Verification items for the finished model (mm, model axes). A direction names the side the tool comes from. Round coordinates to 2 decimals unless told otherwise and drop trailing zeros. Order: outer loops, then holes, each group sorted by start corner. A loop starts at its lowest first (then second) coordinate and runs counter-clockwise, first axis right, second up. Notation, with made-up numbers: M 58.25,-31 L 92.25,-31 A25 ccw 92.25,-3 Z; hole C 40.25,-25 d9. An arc over 180 degrees is marked long. Return JSON: item names as keys, results as strings. Group by question number.
from build123d import *

# Parameters (mm, degrees)
CROQUIS1_R              = 23.4
CROQUIS1_R_2            = 18.4
SALIENTE_EXTRUIR1_DEPTH = 114
CROQUIS2_R              = 23.4
CROQUIS2_R_2            = 7.5
CROQUIS2_R_3            = 1.25
SALIENTE_EXTRUIR2_DEPTH = 5
CORTAR_EXTRUIR1_DEPTH   = 23.5
CROQUIS6_R              = 11.5
CORTAR_EXTRUIR2_DEPTH   = 2.5
CROQUIS9_R              = 2
SALIENTE_EXTRUIR3_DEPTH = 10
REDONDEO3_R             = 10
CROQUIS10_W             = 23.154362093
CROQUIS10_H             = 20
CORTAR_EXTRUIR3_DEPTH   = 10
SALIENTE_EXTRUIR4_DEPTH = 22
REDONDEO1_R             = 10
CROQUIS12_R             = 18.4
CORTAR_EXTRUIR4_DEPTH   = 78


with BuildPart() as part:
    # Croquis1 → Saliente-Extruir1 (new body)
    with BuildSketch(Plane(origin=(0, 0, 0), x_dir=(0, 0, -1), z_dir=(1, 0, 0))):
        Circle(CROQUIS1_R)
        Circle(CROQUIS1_R_2, mode=Mode.SUBTRACT)
    extrude(amount=SALIENTE_EXTRUIR1_DEPTH)

    # Croquis2 → Saliente-Extruir2 (add)
    with BuildSketch(Plane.ZY):
        Circle(CROQUIS2_R)
        Circle(CROQUIS2_R_2, mode=Mode.SUBTRACT)
        with Locations((-11.138131171, -8.481865008)):
            Circle(CROQUIS2_R_3, mode=Mode.SUBTRACT)
        with Locations((8.481865008, -11.138131171)):
            Circle(CROQUIS2_R_3, mode=Mode.SUBTRACT)
        with Locations((11.138131171, 8.481865008)):
            Circle(CROQUIS2_R_3, mode=Mode.SUBTRACT)
        with Locations((-8.481865008, 11.138131171)):
            Circle(CROQUIS2_R_3, mode=Mode.SUBTRACT)
    extrude(amount=-SALIENTE_EXTRUIR2_DEPTH)

    # Croquis4 → Cortar-Extruir1 (cut, symmetric)
    with BuildSketch(Plane.XY):
        Polygon((114, 0.1), (74, -23.4), (114, -23.4), align=None)
    extrude(amount=CORTAR_EXTRUIR1_DEPTH, both=True, mode=Mode.SUBTRACT)

    # Croquis6 → Cortar-Extruir2 (cut)
    with BuildSketch(Plane(origin=(5, 0, 0), x_dir=(0, 0, -1), z_dir=(1, 0, 0))):
        Circle(CROQUIS6_R)
    extrude(amount=-CORTAR_EXTRUIR2_DEPTH, mode=Mode.SUBTRACT)



with BuildPart() as body_2:
    # Croquis9 → Saliente-Extruir3 (new body, symmetric)
    with BuildSketch(Plane.XY):
        Polygon((73.650159213, -43.69341218), (73.650159213, -63.69341218), (53.650159213, -63.69341218), (53.650159213, -43.69341218), (37, -23.4), (59, -23.4), align=None)
        with Locations((58.650159213, -48.69341218)):
            Circle(CROQUIS9_R, mode=Mode.SUBTRACT)
        with Locations((58.650159213, -58.69341218)):
            Circle(CROQUIS9_R, mode=Mode.SUBTRACT)
        with Locations((68.650159213, -58.69341218)):
            Circle(CROQUIS9_R, mode=Mode.SUBTRACT)
        with Locations((68.650159213, -48.69341218)):
            Circle(CROQUIS9_R, mode=Mode.SUBTRACT)
    extrude(amount=SALIENTE_EXTRUIR3_DEPTH, both=True)

    # Redondeo3
    redondeo3_edges = [body_2.edges().sort_by_distance(p)[0] for p in [
        (53.650159213, -43.69341218, 0),
        (73.650159213, -43.69341218, 0),
    ]]
    fillet(redondeo3_edges, radius=REDONDEO3_R)

    # Croquis10 → Cortar-Extruir3 (cut)
    with BuildSketch(Plane.XY.offset(10)):
        with Locations((62.072978167, -53.69341218)):
            Rectangle(CROQUIS10_W, CROQUIS10_H)
    extrude(amount=-CORTAR_EXTRUIR3_DEPTH, mode=Mode.SUBTRACT)


with BuildPart() as part_1:
    add(part.part)

    add(body_2.part)  # Saliente-Extruir4 merges body 2
    # Croquis11 → Saliente-Extruir4 (add)
    with BuildSketch(Plane(origin=(37, 0, 0), x_dir=(0, 0, -1), z_dir=(1, 0, 0))):
        with BuildLine():
            Line((-10, -23.4), (10, -23.4))
            ThreePointArc((10, -23.4), (0, 25.447200239), (-10, -23.4))
        make_face()
    extrude(amount=SALIENTE_EXTRUIR4_DEPTH)

    # Redondeo1
    redondeo1_edges = [part_1.edges().sort_by_distance(p)[0] for p in [
        (48, -23.4, -10),
        (48, -23.4, 10),
    ]]
    fillet(redondeo1_edges, radius=REDONDEO1_R)

    # Croquis12 → Cortar-Extruir4 (cut, through all)
    with BuildSketch(Plane.ZY.offset(-37)):
        Circle(CROQUIS12_R)
    extrude(amount=-CORTAR_EXTRUIR4_DEPTH, mode=Mode.SUBTRACT)


solid = part_1.part
1. Cross-section at D-D (y = 15.5). Enter the section's corners in (x, z).
2. Cross-section at A-A (z = -3). Give the number of separate pieces and of enclosed holes in the cut face, plus the area to 3 significant figures.
3. Cross-section at B-B (z = 22). Enter the section's corners in (x, y), plus the area to 3 significant figures.
4. Access from +Z, -Z, +X, -X, +Y, -Y to the whole of each face (thin tool, end or side, straight path). Record for faces 4 (the face through (18.241, -22.844, 5.073)), 5 (the face through (58, -36, 10)), 6 (the face through (3.8, 11.4, 1.5)).
5. Draft check along X on faces 1 (the face through (56.65, -58.61, -5.07)), 2 (the face through (1.232, 0.33, -7.493)), 3 (the face through (2.5, 0, -8)). Enter one of: +X half, -X half, draft (parallel to the pull), parting line (faces both ways), or undercut.
6. Thickness scan on line 1 along Y through (x, z) = (11, 0.5); line 2 along Z through (x, y) = (15, 0); line 3 along Z through (x, y) = (65.5, -44.5). Record the ranges inside material, lowest first. Write a range as from..to.
7. Go/stop test with flat-tipped pins: pin 1 (8 mm diameter, centred on x = 62, z = 5.5, fed in from -Y); pin 2 (4.5 mm diameter, centred on x = 68.65, y = -58.69, fed in from -Z); pin 3 (1.5 mm diameter, centred on x = 27, z = 5, fed in from -Y). Record where each tip stops, or that it passes through.
8. Cross-section at C-C (x = 11). Enter the section's corners in (y, z), plus the area to 3 significant figures.
Computed:
{
 "1": {"outline": "M 0,-17.53 L 37,-17.53 L 37,-20.18 L 59,-20.18 L 59,-17.53 L 114,-17.53 L 114,-9.92 L 5,-9.92 L 5,9.92 L 114,9.92 L 114,17.53 L 59,17.53 L 59,20.18 L 37,20.18 L 37,17.53 L 0,17.53 Z"},
 "2": {"separate pieces": "2", "enclosed holes": "4", "area": "1,890 mm²"},
 "3": {"outline": "M 0,-7.97 L 37,-7.97 L 37,-12.79 L 59,-12.79 L 59,-7.97 L 100.26,-7.97 L 114,0.1 L 114,7.97 L 59,7.97 L 59,12.79 L 37,12.79 L 37,7.97 L 0,7.97 Z", "area": "1,970 mm²"},
 "4": {"face 4": "-X", "face 5": "+Z, +X, -X, -Y", "face 6": "+X"},
 "5": {"face 1": "undercut", "face 2": "draft", "face 3": "+X half"},
 "6": {"line 1": "y = -23.39..-18.39, 18.39..23.39", "line 2": "z = -23.4..-18.4, 18.4..23.4", "line 3": "z = -10..0"},
 "7": {"pin 1": "stops at y = -43.69", "pin 2": "stops at z = -10", "pin 3": "stops at y = -23.01"},
 "8": {"outline": "C 0,0 d46.8; hole C 0,0 d36.8", "area": "657 mm²"}
}
